Answer from the drawing. Dimensions are ordinates in mm from the lowest x, y and z of the part. A direction names the side the tool comes from. Round coordinates to 2 decimals unless told otherwise and drop trailing zeros. Order: outer loops, then holes, each group sorted by start corner. A loop starts at its lowest first (then second) coordinate and runs counter-clockwise, first axis right, second up. Notation, with made-up numbers: (19.5, 78) -> (55.5, 78) arc R22 ccw to (55.5, 104) -> close; hole circle Ø8 at (9.25, -16.5). An arc over 180 degrees is marked (long way). Use a Markdown table: item, result. Add a question column.
1. Section A-A, the plane z = 66 is taken. Give the vertices of the cut face in (x, y).
2. Given pin 1 (21.5 mm diameter, centred on x = 63.5, y = 27.5, fed in from +Z); pin 2 (1 mm diameter, centred on y = 11.5, z = 29.5, fed in from -X); pin 3 (8 mm diameter, centred on x = 100, z = 60, fed in from +Y), each flat-ended and moving along its own axis, determine where each tip first touches the part or whether it passes through.
3. Section C-C, the plane x = 61.5 is taken. Give the vertices of the cut face in (y, z).
4. Section B-B, the plane y = 18 is taken. Give the vertices of the cut face in (x, z).
5. Consider L1, parallel to X at y = 6, z = 43.5; L2, parallel to Y at x = 117, z = 26. Determine where each line is inside the solid, lowest interval first. Write a range as [from, to].
6. For the marked faces 1 and 2, determine the directions among +Z, -Z, +X, -X, +Y, -Y from which every point of the face is accessible in a straight line to the end or side of a thin tool.
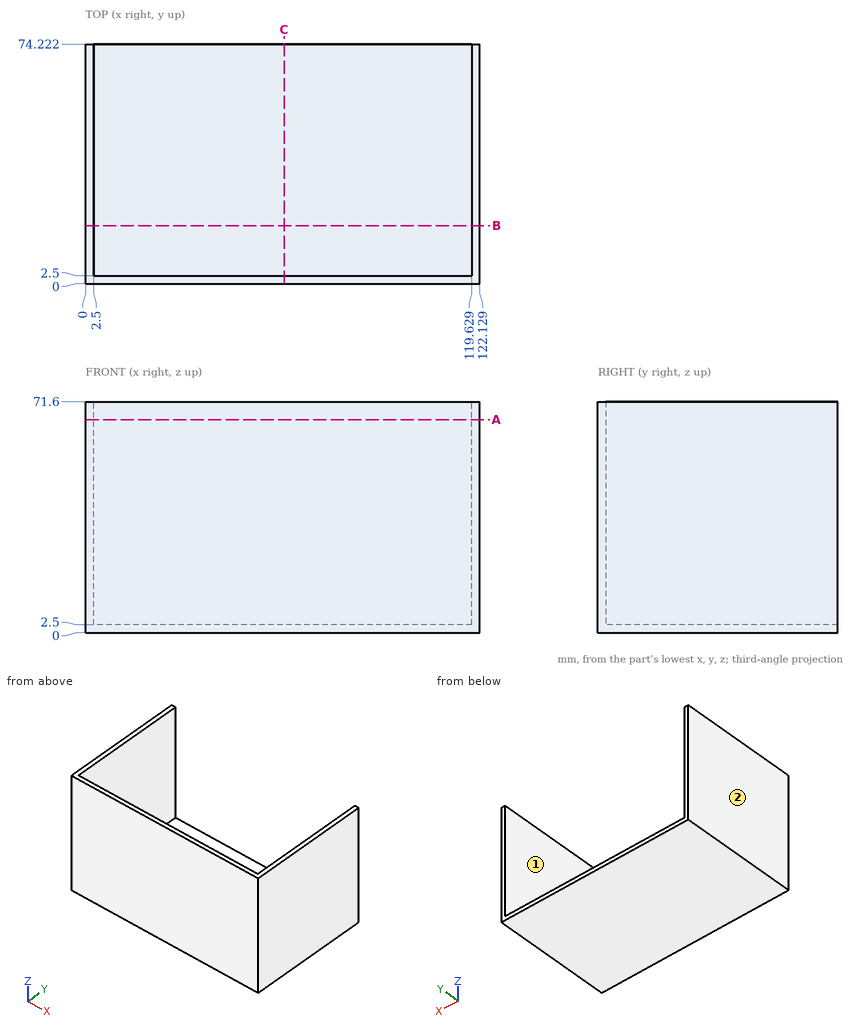
Verdict:
| question | item | result |
|---|---|---|
| 1 | outline | (0, 0) -> (122.13, 0) -> (122.13, 74.22) -> (119.63, 74.22) -> (119.63, 2.5) -> (2.5, 2.5) -> (2.5, 74.22) -> (0, 74.22) -> close |
| 2 | pin 1 | stops at z = 2.5 |
| 2 | pin 2 | stops at x = 0 |
| 2 | pin 3 | stops at y = 2.5 |
| 3 | outline | (0, 0) -> (74.22, 0) -> (74.22, 2.5) -> (2.5, 2.5) -> (2.5, 71.6) -> (0, 71.6) -> close |
| 4 | outline | (0, 0) -> (122.13, 0) -> (122.13, 71.6) -> (119.63, 71.6) -> (119.63, 2.5) -> (2.5, 2.5) -> (2.5, 71.6) -> (0, 71.6) -> close |
| 5 | L1 | x = [0, 2.5], [119.63, 122.13] |
| 5 | L2 | y = [0, 2.5] |
| 6 | face 1 | +Z, +Y |
| 6 | face 2 | +Z, -Z, -X, +Y, -Y |
